Autodesk Inventor part; units mm, degrees
ref_plane "YZ Plane" through (0, 0, 0) normal (1, 0, 0) x (0, 1, 0)
ref_plane "XZ Plane" through (0, 0, 0) normal (0, 1, 0) x (-1, 0, 0)
ref_plane "XY Plane" through (0, 0, 0) normal (0, 0, 1) x (1, 0, 0)
sketch "Sketch1" plane through (0, 0, 0) normal (0, 1, 0) x (-1, 0, 0)
  circle A0 centre (-20, 47.5) radius 1.6
  circle A1 centre (20, 47.5) radius 1.6
  circle A2 centre (-20, -92.5) radius 1.6
  circle A3 centre (20, -92.5) radius 1.6
  line L0 (20, 55) -> (-20, 55)
  line L1 (-25, -92.5) -> (-25, -92.5494)
  line L2 (25, -92.5) -> (25, -92.5494)
  arc A4 (-21.0561, -97.4366) -> (21.0561, -97.4366) centre (0, 0) ccw
  arc A5 (21.0561, -97.4366) -> (25, -92.5494) centre (20, -92.5494) ccw
  arc A6 (-25, -92.5494) -> (-21.0561, -97.4366) centre (-20, -92.5494) ccw
  arc A7 (-20, 55) -> (-25, 50) centre (-20, 50) ccw
  arc A8 (25, 50) -> (20, 55) centre (20, 50) ccw
  circle A9 centre (-10.5, -49.6569) radius 1.65
  circle A10 centre (10.5, -49.6569) radius 1.6
  circle A11 centre (-12.5, -72.5) radius 6.25
  circle A12 centre (12.5, -72.5) radius 6.25
  line L3 (-20, 38.3431) -> (-20, -38)
  line L4 (-24.4142, 43.5858) -> (-20.5858, 39.7574)
  line L5 (-24.4142, -43.2426) -> (-20.5858, -39.4142)
  line L6 (-25, -92.5494) -> (-25, -44.6569)
  line L7 (-25, 45) -> (-25, 50)
  line L8 (20, 38.3431) -> (20, -38)
  line L9 (24.4142, 43.5858) -> (20.5858, 39.7574)
  line L10 (24.4142, -43.2426) -> (20.5858, -39.4142)
  line L11 (25, -92.5494) -> (25, -44.6569)
  line L12 (25, 45) -> (25, 50)
  arc A13 (-25, 45) -> (-24.4142, 43.5858) centre (-23, 45) ccw
  arc A14 (-20, 38.3431) -> (-20.5858, 39.7574) centre (-22, 38.3431) ccw
  arc A15 (-20.5858, -39.4142) -> (-20, -38) centre (-22, -38) ccw
  arc A16 (-24.4142, -43.2426) -> (-25, -44.6569) centre (-23, -44.6569) ccw
  arc A17 (25, -44.6569) -> (24.4142, -43.2426) centre (23, -44.6569) ccw
  arc A18 (20, -38) -> (20.5858, -39.4142) centre (22, -38) ccw
  arc A19 (20.5858, 39.7574) -> (20, 38.3431) centre (22, 38.3431) ccw
  arc A20 (24.4142, 43.5858) -> (25, 45) centre (23, 45) ccw
extrude "Extrusion1" add sketch "Sketch1" along normal blind 3
properties part number "Top Plate" material "Polycarbonate, Clear"
The model under review builds one solid part; all positions refer to its coordinate system, in mm. A direction names the side the tool comes from. Round coordinates to 2 decimals unless told otherwise and drop trailing zeros. Write each loop counter-clockwise with the first axis right and the second up, starting at its lowest first coordinate (ties: lowest second). Pieces come first, ordered by that corner, then holes.
(1) We need section D-D on z = 10.5. Give the boundary of the cut face in (x, y), and give its area (3 significant figures).
(2) Wall thickness on L1, parallel to X at y = 2, z = -92.5; L2, parallel to Z at x = 10.5, y = 1.5; L3, parallel to Z at x = 11.5, y = 0.6: over which ranges is each line inside the solid? List them lowest first.
(3) We need section C-C on y = 0.8. Give the number of separate pieces and of enclosed holes in the cut face, and give its area (3 significant figures).
(4) We need section B-B on x = 10.5. Give the boundary of the cut face in (y, z), and give its area (3 significant figures).
(5) Mouldability with a two-part tool opening along Z and no side actions: class faces 1 (the cylindrical face through (-10.292, 1.479, -51.243)), 2 (the cylindrical face through (-0.297, 1.479, -99.685)), 3 (the flat face through (0, 1, 55)) as +Z half, -Z half, draft (parallel to the pull), parting line (faces both ways), or undercut.
(6) We need section A-A on z = 47.5. Give the boundary of the cut face in (x, y).
(7) Machinability: for faces 4 (the cylindrical face through (19.26, 1.48, 48.92)), 5 (the flat face through (-20, 1, 1)), 6 (the flat face through (20, 1, 1)), which of the approach directions +Z, -Z, +X, -X, +Y, -Y give a long, thin tool a straight path to every point of the face, cutting with its end or side? Answer none if there is none.
(8) Insertion check: pin 1 (3 mm diameter, centred on x = -20, z = 47.5, fed in from -Y); pin 2 (0.9 mm diameter, centred on y = 1, z = 9, fed in from -X); pin 3 (1.5 mm diameter, centred on y = 1.5, z = -9.5, fed in from +X). Each pin has a flat end and moves straight along its axis. Give the tip position at first contact, or say it passes through.
Findings below:
1. outline: (-20, 0) - (20, 0) - (20, 3) - (-20, 3) - close
1. area: 120 mm2
2. L1: x = -25 to -21.6, -18.4 to 18.4, 21.6 to 25
2. L2: z = -99.13 to -78.42, -66.58 to -51.31, -48.01 to 55
2. L3: z = -99.02 to -78.67, -66.33 to -50.97, -48.34 to 55
3. separate pieces: 1
3. enclosed holes: 8
3. area: 6,540 mm2
4. outline: (0, -99.13) - (3, -99.13) - (3, -78.42) - (0, -78.42) - close; (0, -66.58) - (3, -66.58) - (3, -51.31) - (0, -51.31) - close; (0, -48.01) - (3, -48.01) - (3, 55) - (0, 55) - close
4. area: 417 mm2
5. face 1: undercut
5. face 2: -Z half
5. face 3: +Z half
6. outline: (-25, 0) - (-21.6, 0) - (-21.6, 3) - (-25, 3) - close; (-18.4, 0) - (18.4, 0) - (18.4, 3) - (-18.4, 3) - close; (21.6, 0) - (25, 0) - (25, 3) - (21.6, 3) - close
7. face 4: +Y, -Y
7. face 5: -X, +Y, -Y
7. face 6: +X, +Y, -Y
8. pin 1: passes through
8. pin 2: stops at x = -20
8. pin 3: stops at x = 20
